Can you work these out from the model? Positions are in its coordinate system, mm. A direction names the side the tool comes from. Coordinates: 2 decimals unless noted, no trailing zeros. Order: outer loops, then holes, each group sorted by start corner. A loop starts at its lowest first (then second) coordinate and runs counter-clockwise, first axis right, second up. Notation, with made-up numbers: (69, 76) - (124, 76) arc R28 ccw to (124, 105) - close; hole circle Ø9 at (80.5, -11). An arc over 180 degrees is marked (long way). Return JSON: item names as keys, results as strings. Group by question number.
1) Imagine slicing it at C-C (z = 15). Write out the boundary of the cut face in (x, y).
2) If we mould it in two halves opening along X, with no side actions, what happens to faces 1 (the face through (2, 44.3, 8.6)), 2 (the face through (12.142, 39.494, 2.465)), 3 (the face through (13.403, 11.534, 2.465)), 4 (the face through (6.175, 15.255, 21.794))? For each: pulls with the +X half, pulls with the -X half, needs draft (parallel to the pull), parting line crosses it, or undercut.
3) Imagine slicing it at B-B (y = 40). Write out the boundary of the cut face in (x, z), and give its area (3 significant figures).
4) Imagine slicing it at D-D (z = 33). Write out the boundary of the cut face in (x, y).
5) Imagine slicing it at A-A (x = 5.5). Write out the boundary of the cut face in (y, z), and give its area (3 significant figures).
6) Which directions (+Z, -Z, +X, -X, +Y, -Y) give clear straight access to the entire face, cutting with the end or side of a thin tool? Please do faces 5 (the face through (8, 23, 18)), 6 (the face through (0, 5, 19)), 7 (the face through (21.3, 38, 2)), 8 (the face through (0, 40, 11)).
7) If I drill on line 1 along X through (y, z) = (9.65, 3.1); line 2 along Z through (x, y) = (5, 15); line 3 along X through (y, z) = (9, 1), over which ranges is the centre line in solid material (lowest first)?
8) For pin 1 Ø10 at (x, z) = (7.5, 33) entering from +Y; pin 2 Ø1.5 at (x, z) = (42.5, 10.5) entering from +Y; pin 3 Ø13.5 at (y, z) = (15, 16) entering from -X; pin 4 Ø6.5 at (x, y) = (4, 27) entering from +Z, each with a flat end and sliding along its axis, tell me the tip position at first contact or that it passes through.
```python
from build123d import *

# Parameters (mm, degrees)
CYLINDER002_R           = 3.05
CYLINDER002_DEPTH       = 10
CYLINDER004_R           = 1.9
CYLINDER004_DEPTH       = 20
CYLINDER005_R           = 1.9
CYLINDER005_DEPTH       = 20
CYLINDER003_R           = 1.9
CYLINDER003_DEPTH       = 20
CYLINDER006_R           = 11.8
CYLINDER006_DEPTH       = 10
CYLINDER001_R           = 5.8
CYLINDER001_DEPTH       = 10
CUBE004_W               = 10
CUBE004_H               = 70
CUBE004_DEPTH           = 40
CUBE005_W               = 40
CUBE005_H               = 40
CUBE005_DEPTH           = 10
CUBE006_W               = 15
CUBE006_H               = 15
CUBE006_DEPTH           = 10
CUBE007_W               = 10
CUBE007_H               = 10
CUBE007_DEPTH           = 10
CUBE007_PLACEMENT_ANGLE = 45
CUBE008_W               = 10
CUBE008_H               = 10
CUBE008_DEPTH           = 10
CUBE008_PLACEMENT_ANGLE = 45
CUBE009_W               = 10
CUBE009_H               = 20
CUBE009_DEPTH           = 10
CUBE010_W               = 10
CUBE010_H               = 40
CUBE010_DEPTH           = 40
CUBE010_PLACEMENT_ANGLE = 45
CUBE011_W               = 10
CUBE011_H               = 10
CUBE011_DEPTH           = 39
CUBE011_PLACEMENT_ANGLE = 45
CYLINDER_R              = 3.5
CYLINDER_DEPTH          = 39
CUBE003_W               = 10
CUBE003_H               = 70
CUBE003_DEPTH           = 40
CUBE003_ROLL_ANGLE      = -34.999976
CUBE003_PLACEMENT_ANGLE = -90
CUBE002_W               = 4
CUBE002_H               = 8
CUBE002_DEPTH           = 39
CUBE001_W               = 60
CUBE001_H               = 60
CUBE001_DEPTH           = 60
CUBE_W                  = 50.3
CUBE_H                  = 46.3
CUBE_DEPTH              = 39


with BuildPart() as cylinder002:
    # cylinder002 → cylinder002 (new body)
    with BuildSketch(Plane(origin=(-3, 15, 16), x_dir=(0, 0, -1), z_dir=(1, 0, 0))):
        Circle(CYLINDER002_R)
    extrude(amount=CYLINDER002_DEPTH)


with BuildPart() as cylinder004:
    # cylinder004 → cylinder004 (new body)
    with BuildSketch(Plane(origin=(31, 0, -0.1), x_dir=(1, 0, 0), z_dir=(0, 0, 1))):
        Circle(CYLINDER004_R)
    extrude(amount=CYLINDER004_DEPTH)


with BuildPart() as cylinder005:
    # cylinder005 → cylinder005 (new body)
    with BuildSketch(Plane(origin=(0, 31, -0.1), x_dir=(1, 0, 0), z_dir=(0, 0, 1))):
        Circle(CYLINDER005_R)
    extrude(amount=CYLINDER005_DEPTH)


with BuildPart() as matrix_union:
    # cylinder003 → cylinder003 (new body)
    with BuildSketch(Plane.XY.offset(-0.1)):
        Circle(CYLINDER003_R)
    extrude(amount=CYLINDER003_DEPTH)

    # Matrix_Union: union cylinder004, cylinder005
    add(cylinder004.part)
    add(cylinder005.part)


with BuildPart() as matrix_union_1:
    # Matrix_Union placement: moved
    add(matrix_union.part.moved(Location((13.65, 9.65, -0.1))))


with BuildPart() as cylinder006:
    # cylinder006 → cylinder006 (new body)
    with BuildSketch(Plane(origin=(29.3, 25.3, -0.1), x_dir=(1, 0, 0), z_dir=(0, 0, 1))):
        Circle(CYLINDER006_R)
    extrude(amount=CYLINDER006_DEPTH)


with BuildPart() as group002:
    # cylinder001 → cylinder001 (new body)
    with BuildSketch(Plane(origin=(4.4, 15, 16), x_dir=(0, 0, -1), z_dir=(1, 0, 0))):
        Circle(CYLINDER001_R)
    extrude(amount=CYLINDER001_DEPTH)

    # Group002: union cylinder002, Matrix_Union, cylinder006
    add(cylinder002.part)
    add(matrix_union_1.part)
    add(cylinder006.part)


with BuildPart() as cube004:
    # cube004 → cube004 (new body)
    with BuildSketch(Plane(origin=(8, 5, 36.5), x_dir=(0, -1, 0), z_dir=(0, 0, 1))):
        with Locations((5, 35)):
            Rectangle(CUBE004_W, CUBE004_H)
    extrude(amount=CUBE004_DEPTH)


with BuildPart() as cube005:
    # cube005 → cube005 (new body)
    with BuildSketch(Plane(origin=(21.3, 17.3, -0.1), x_dir=(1, 0, 0), z_dir=(0, 0, 1))):
        with Locations((20, 20)):
            Rectangle(CUBE005_W, CUBE005_H)
    extrude(amount=CUBE005_DEPTH)


with BuildPart() as cube006:
    # cube006 → cube006 (new body)
    with BuildSketch(Plane(origin=(34.3, 15.3, -0.1), x_dir=(1, 0, 0), z_dir=(0, 0, 1))):
        with Locations((7.5, 7.5)):
            Rectangle(CUBE006_W, CUBE006_H)
    extrude(amount=CUBE006_DEPTH)


with BuildPart() as cube007:
    # cube007 → cube007 (new body)
    with BuildSketch(Plane.XY):
        with Locations((5, 5)):
            Rectangle(CUBE007_W, CUBE007_H)
    extrude(amount=CUBE007_DEPTH)


with BuildPart() as cube007_1:
    # cube007 placement: moved
    add(cube007.part.moved(Location((50.3, 13, -0.1))).rotate(Axis((50.3, 13, -0.1), (0, 0, 1)), CUBE007_PLACEMENT_ANGLE))


with BuildPart() as cube008:
    # cube008 → cube008 (new body)
    with BuildSketch(Plane.XY):
        with Locations((5, 5)):
            Rectangle(CUBE008_W, CUBE008_H)
    extrude(amount=CUBE008_DEPTH)


with BuildPart() as cube008_1:
    # cube008 placement: moved
    add(cube008.part.moved(Location((17, 46.3, -0.1))).rotate(Axis((17, 46.3, -0.1), (0, 0, -1)), CUBE008_PLACEMENT_ANGLE))


with BuildPart() as cube009:
    # cube009 → cube009 (new body)
    with BuildSketch(Plane(origin=(-0.1, 20.3, 29.5), x_dir=(1, 0, 0), z_dir=(0, 0, 1))):
        with Locations((5, 10)):
            Rectangle(CUBE009_W, CUBE009_H)
    extrude(amount=CUBE009_DEPTH)


with BuildPart() as cube010:
    # cube010 → cube010 (new body)
    with BuildSketch(Plane.XY):
        with Locations((5, 20)):
            Rectangle(CUBE010_W, CUBE010_H)
    extrude(amount=CUBE010_DEPTH)


with BuildPart() as cube010_1:
    # cube010 placement: moved
    add(cube010.part.moved(Location((-0.1, 30.3, 29.5))).rotate(Axis((-0.1, 30.3, 29.5), (-1, 0, 0)), CUBE010_PLACEMENT_ANGLE))


with BuildPart() as cube011:
    # cube011 → cube011 (new body)
    with BuildSketch(Plane.XY):
        with Locations((5, 5)):
            Rectangle(CUBE011_W, CUBE011_H)
    extrude(amount=CUBE011_DEPTH)


with BuildPart() as cube011_1:
    # cube011 placement: moved
    add(cube011.part.moved(Location((0, 42.3, -0.1))).rotate(Axis((0, 42.3, -0.1), (0, 0, 1)), CUBE011_PLACEMENT_ANGLE))


with BuildPart() as cylinder:
    # cylinder → cylinder (new body)
    with BuildSketch(Plane(origin=(0, 33.5, -0.1), x_dir=(1, 0, 0), z_dir=(0, 0, 1))):
        Circle(CYLINDER_R)
    extrude(amount=CYLINDER_DEPTH)


with BuildPart() as union:
    # cube003 → cube003 (new body)
    with BuildSketch(Plane.XY):
        with Locations((5, 35)):
            Rectangle(CUBE003_W, CUBE003_H)
    extrude(amount=CUBE003_DEPTH)


with BuildPart() as union_1:
    # cube003 roll: moved
    add(union.part.rotate(Axis((0, 0, 0), (1, 0, 0)), CUBE003_ROLL_ANGLE))


with BuildPart() as union_2:
    # cube003 placement: moved
    add(union_1.part.moved(Location((8, 5, 36.5))).rotate(Axis((8, 5, 36.5), (0, 0, 1)), CUBE003_PLACEMENT_ANGLE))

    # Group001: union cube004, cube005, cube006, cube007, cube008, cube009, cube010, cube011, cylinder
    add(cube004.part)
    add(cube005.part)
    add(cube006.part)
    add(cube007_1.part)
    add(cube008_1.part)
    add(cube009.part)
    add(cube010_1.part)
    add(cube011_1.part)
    add(cylinder.part)

    # union: union Group002
    add(group002.part)


with BuildPart() as cube002:
    # cube002 → cube002 (new body)
    with BuildSketch(Plane(origin=(-2, 11, 0), x_dir=(1, 0, 0), z_dir=(0, 0, 1))):
        with Locations((2, 4)):
            Rectangle(CUBE002_W, CUBE002_H)
    extrude(amount=CUBE002_DEPTH)


with BuildPart() as cube001:
    # cube001 → cube001 (new body)
    with BuildSketch(Plane(origin=(8, 4, 5), x_dir=(1, 0, 0), z_dir=(0, 0, 1))):
        with Locations((30, 30)):
            Rectangle(CUBE001_W, CUBE001_H)
    extrude(amount=CUBE001_DEPTH)


with BuildPart() as difference001:
    # cube → cube (new body)
    with BuildSketch(Plane.XY):
        with Locations((25.15, 23.15)):
            Rectangle(CUBE_W, CUBE_H)
    extrude(amount=CUBE_DEPTH)

    # difference: cut cube001
    add(cube001.part, mode=Mode.SUBTRACT)

    # Group: union cube002
    add(cube002.part)

    # difference001: cut union
    add(union_2.part, mode=Mode.SUBTRACT)


solid = difference001.part
```
Calculated:
{
 "1": {"outline": "(-2, 11) - (0, 11) - (0, 0) - (38.71, 0) - (38.71, 4) - (8, 4) - (8, 9.29) - (4.4, 9.29) - (4.4, 12.12) - (-2, 12.12) - close; (-2, 17.88) - (4.4, 17.88) - (4.4, 20.71) - (8, 20.71) - (8, 44.8) - (2.5, 44.8) - (0, 42.3) - (0, 37) arc R3.5 cw to (0, 30) - (0, 19) - (-2, 19) - close"},
 "2": {"face 1": "pulls with the -X half", "face 2": "undercut", "face 3": "undercut", "face 4": "needs draft"},
 "3": {"outline": "(0, 0) - (11.86, 0) - (11.86, 5) - (8, 5) - (8, 19.8) - (0, 19.8) - close; (15.44, 0) - (21.3, 0) - (21.3, 5) - (15.44, 5) - close", "area": "207 mm2"},
 "4": {"outline": "(-2, 11) - (0, 11) - (0, 0) - (13, 0) - (13, 4) - (8, 4) - (8, 20.3) - (0, 20.3) - (0, 19) - (-2, 19) - close"},
 "5": {"outline": "(0, 0) - (46.3, 0) - (46.3, 13.5) - (30.3, 29.5) - (20.3, 29.5) - (20.3, 39) - (0, 39) - close; hole circle Ø11.6 at (15, 16)", "area": "1,330 mm2"},
 "6": {"face 5": "+Z, +X, +Y", "face 6": "+Z, -Z, -X, -Y", "face 7": "+Z, -Z, +X, +Y", "face 8": "+Z, -Z, -X, +Y"},
 "7": {"line 1": "0 to 11.75, 15.55 to 42.75, 46.55 to 50.3", "line 2": "0 to 10.2, 21.8 to 39", "line 3": "0 to 11.86, 15.44 to 42.86, 46.44 to 50.3"},
 "8": {"pin 1": "y = 31.8", "pin 2": "y = 4", "pin 3": "x = -2", "pin 4": "z = 29.5"}
}
